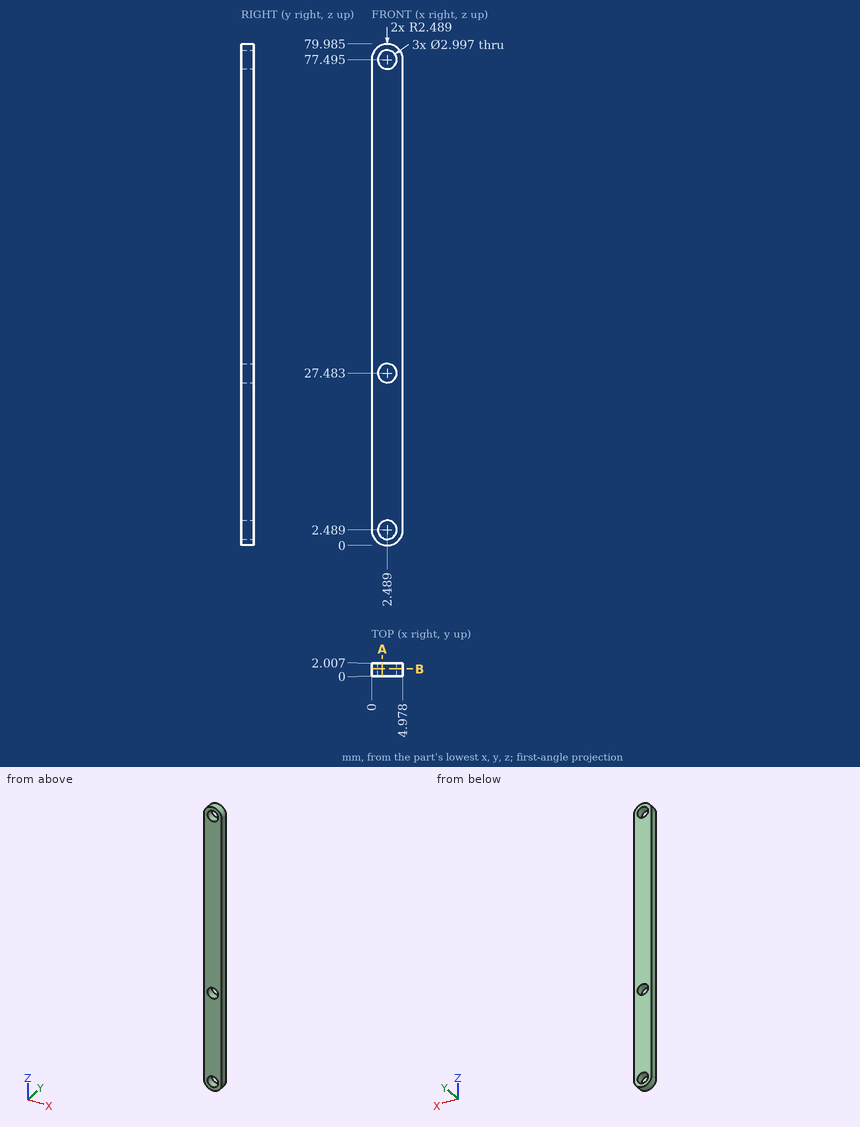
The figure shows three views and two pictorial views of one solid part (mm, origin at its lowest corner). Answer the questions. Coordinates: 2 decimals unless noted, no trailing zeros. Loops run counter-clockwise (first coordinate to the right, second up) from the corner with the lowest first, then second, coordinate; pieces in that order, holes last.
(1) Consider line 1 along Z through (x, y) = (3.4, 1.2) (1 decimal); line 2 along Z through (x, y) = (3.85, 0.85) (1 decimal); line 3 along Z through (x, y) = (0.5, 0.6) (1 decimal). Determine where each line is inside the solid, lowest interval first.
Solution:
line 1: z = 0.2 to 1.3, 3.7 to 26.3, 28.7 to 76.3, 78.7 to 79.8
line 2: z = 0.4 to 1.9, 3.1 to 26.9, 28.1 to 76.9, 78.1 to 79.6
line 3: z = 1 to 79
(2) A flat-ended cylindrical pin translates along its axis: pin 1 Ø2.5 at (x, z) = (2.49, 27.48) entering from +Y. Find the tip coordinate at first contact, or state that the pin passes through.
Solution:
pin 1: passes through
(3) The part is cut by section B-B (y = 1.15). Determine the outline of the cut face in (x, z) (1 decimal).
Solution:
outline: (0, 2.5) arc R2.5 ccw to (5, 2.5) - (5, 77.5) arc R2.5 ccw to (0, 77.5) - close; hole circle Ø3 at (2.5, 2.5); hole circle Ø3 at (2.5, 27.5); hole circle Ø3 at (2.5, 77.5)
(4) The part is cut by section A-A (x = 1.7). Determine the outline of the cut face in (y, z) (1 decimal), and give its area (3 significant figures).
Solution:
outline: (0, 0.1) - (2, 0.1) - (2, 1.2) - (0, 1.2) - close; (0, 3.8) - (2, 3.8) - (2, 26.2) - (0, 26.2) - close; (0, 28.8) - (2, 28.8) - (2, 76.2) - (0, 76.2) - close; (0, 78.8) - (2, 78.8) - (2, 79.9) - (0, 79.9) - close
area: 145 mm2
